The model under review builds one solid part; all positions refer to its coordinate system, in mm. A direction names the side the tool comes from. Coordinates: 2 decimals unless noted, no trailing zeros. Loops run counter-clockwise (first coordinate to the right, second up) from the corner with the lowest first, then second, coordinate; pieces in that order, holes last. Notation, with made-up numbers: M -10,-13 L 13,-13 A37 ccw 13,26 Z; hole C 11.25,17 d5. An arc over 180 degrees is marked long. Return JSON: item names as keys, results as strings.
```python
from build123d import *

# Parameters (mm, degrees)
F0_W      = 52
F0_H      = 15
F1_DEPTH  = 45
F2_DEPTH  = 61
F3_R      = 22.5
F4_DEPTH  = 15
F6_R      = 9
F5_R      = 9
F7_DEPTH  = 25
F10_DEPTH = 25


with BuildPart() as f1:
    # F0 (on Front) → F1 (new body)
    with BuildSketch(Plane.XZ):
        with Locations((-56.5, -7.6666666667)):
            Rectangle(F0_W, F0_H)
    extrude(amount=F1_DEPTH)



with BuildPart() as f1b:
    # F0 (on Front) → F1, piece 2 (new body)
    with BuildSketch(Plane.XZ):
        with Locations((56.5, -7.6666666667)):
            Rectangle(F0_W, F0_H)
    extrude(amount=F1_DEPTH)


with BuildPart() as f1_1:
    add(f1.part)

    add(f1b.part)  # F2 merges F1b
    # F0 (on Front) → F2 (join)
    with BuildSketch(Plane.XZ):
        Polygon((30.5, 45.8333333333), (-30.5, 45.8333333333), (-30.5, -0.1666666667), (-30.5, -15.1666666667), (30.5, -15.1666666667), (30.5, -0.1666666667), align=None)
    extrude(amount=F2_DEPTH)

    # F3 (on face) → F4 (join)
    with BuildSketch(Plane.XY.offset(-0.1666666667)):
        with BuildLine():
            Line((-82.5, -45), (-82.5, 0))
            ThreePointArc((-82.5, 0), (-105, -22.5), (-82.5, -45))
        make_face()
        with Locations((82.5, -22.5)):
            Circle(F3_R)
    extrude(amount=-F4_DEPTH)

    # F6 (on face) + F5 (on face) → F7 (cut)
    with BuildSketch(Plane.XY.offset(-0.1666666667)):
        with Locations((82.5, -22.5)):
            Circle(F6_R)
    with BuildSketch(Plane.XY.offset(-0.1666666667)):
        with Locations((-82.5, -22.5)):
            Circle(F5_R)
    extrude(amount=-F7_DEPTH, mode=Mode.SUBTRACT)

    # F9 (on offset) → F10 (cut)
    with BuildSketch(Plane(origin=(-15, 0, 0), x_dir=(0, -1, 0), z_dir=(-1, 0, 0))):
        Polygon((61.0416666667, 45.8333333333), (10.7916666667, 45.8333333333), (50.0416666667, -15.1666666667), (61.0416666667, -15.1666666667), align=None)
    extrude(amount=-F10_DEPTH, mode=Mode.SUBTRACT)


solid = f1_1.part
```
1. Add section B-B on y = -22.5. Give the boundary of the cut face in (x, z), plus the area to 3 significant figures.
Check values:
{"outline": "M -105,-15.17 L -91.5,-15.17 L -91.5,-0.17 L -105,-0.17 Z; M -73.5,-15.17 L 73.5,-15.17 L 73.5,-0.17 L 30.5,-0.17 L 30.5,45.83 L 10,45.83 L 10,27.64 L -15,27.64 L -15,45.83 L -30.5,45.83 L -30.5,-0.17 L -73.5,-0.17 Z; M 91.5,-15.17 L 105,-15.17 L 105,-0.17 L 91.5,-0.17 Z", "area": "4,960 mm²"}
2. The part is to be moulded in two halves that separate along X. For faces 5 (the face through (-104.995, -22.005, -7.562)), 6 (the face through (-2.68, -30.14, 15.76)), 7 (the face through (-73.916, -19.797, -7.562)), 8 (the face through (-23, -61, 16)), say which applies: released by +X, released by -X, zero draft, split by the parting line, or undercut.
Check values:
{"face 5": "released by -X", "face 6": "undercut", "face 7": "undercut", "face 8": "zero draft"}
3. Add section A-A on z = -10. Give the boundary of the cut face in (x, y), plus the area to 3 significant figures.
Check values:
{"outline": "M -82.5,-45 L -30.5,-45 L -30.5,-61 L -15,-61 L -15,-46.72 L 10,-46.72 L 10,-61 L 30.5,-61 L 30.5,-45 L 82.5,-45 A22.5 ccw 82.5,0 L -82.5,0 A22.5 ccw Z; hole C -82.5,-22.5 d18; hole C 82.5,-22.5 d18", "area": "9,130 mm²"}
4. To check wall thickness, follow line 1 (X direction, y = -22, z = -11); line 2 (Y direction, x = -82.5, z = -10.5); line 3 (X direction, y = -44.5, z = 15). State the ranges of each line that lie inside material, in increasing order.
Check values:
{"line 1": "-104.99 to -91.49, -73.51 to 73.51, 91.49 to 104.99", "line 2": "-45 to -31.5, -13.5 to 0", "line 3": "-30.5 to -15, 10 to 30.5"}
5. Insertion check: pin 1 Ø13.5 at (x, y) = (64, -31) entering from +Z; pin 2 Ø4 at (y, z) = (-16.5, 10.5) entering from +X; pin 3 Ø18.5 at (y, z) = (-35.5, 20) entering from -X. Each pin has a flat end and moves straight along its axis. Give the tip position at first contact, or say it passes through.
Check values:
{"pin 1": "z = -0.17", "pin 2": "x = 30.5", "pin 3": "x = -30.5"}
6. Add section C-C on x = 89. Give the boundary of the cut face in (y, z).
Check values:
{"outline": "M -44.04,-15.17 L -28.72,-15.17 L -28.72,-0.17 L -44.04,-0.17 Z; M -16.28,-15.17 L -0.96,-15.17 L -0.96,-0.17 L -16.28,-0.17 Z"}
7. Add section D-D on z = 16.5. Give the boundary of the cut face in (x, y), plus the area to 3 significant figures.
Check values:
{"outline": "M -30.5,-61 L -15,-61 L -15,-29.67 L 10,-29.67 L 10,-61 L 30.5,-61 L 30.5,0 L -30.5,0 Z", "area": "2,940 mm²"}
8. Machinability: for faces 1 (the face through (67, -22, -0.167)), 2 (the face through (-68, -22, -0.167)), 3 (the face through (-15, -41, 23)), 4 (the face through (56, -45, -8)), which of the approach directions +Z, -Z, +X, -X, +Y, -Y give a long, thin tool a straight path to every point of the face, cutting with its end or side? Answer none if there is none.
Check values:
{"face 1": "+Z, +X, +Y, -Y", "face 2": "+Z, -X, +Y, -Y", "face 3": "+Z, -Y", "face 4": "+Z, -Z, +X, -Y"}
